Here's how the part is built. I have some questions about the finished solid (model axes, mm). A direction names the side the tool comes from. Coordinates: 2 decimals unless noted, no trailing zeros. Write each loop counter-clockwise with the first axis right and the second up, starting at its lowest first coordinate (ties: lowest second). Pieces come first, ordered by that corner, then holes.
```python
from build123d import *

# Parameters (mm, degrees)
BOSS_EXTRUDE1_DEPTH = 30
SKETCH2_R           = 11
CUT_EXTRUDE1_DEPTH  = 60
FILLET1_R           = 10
SKETCH3_R           = 2
CUT_EXTRUDE2_DEPTH  = 10
SKETCH13_R          = 13.5
CUT_EXTRUDE3_DEPTH  = 10


with BuildPart() as part:
    # Sketch1 → Boss-Extrude1 (new body, symmetric)
    with BuildSketch(Plane.XY):
        Polygon((-30, 30), (-30, -30), (30, -30), (30, 30), (24, 30), (24, -24.147945483), (-20, -24.147945483), (-20, 30), align=None)
    extrude(amount=BOSS_EXTRUDE1_DEPTH, both=True)

    # Sketch2 → Cut-Extrude1 (cut)
    with BuildSketch(Plane(origin=(0, 0, 0), x_dir=(0, 0, -1), z_dir=(1, 0, 0))):
        Circle(SKETCH2_R)
    extrude(amount=-CUT_EXTRUDE1_DEPTH, mode=Mode.SUBTRACT)

    # Fillet1
    fillet1_edges = [part.edges().sort_by_distance(p)[0] for p in [
        (-25, 30, -30),
        (27, 30, 30),
        (-25, 30, 30),
        (27, 30, -30),
    ]]
    fillet(fillet1_edges, radius=FILLET1_R)

    # Sketch3 → Cut-Extrude2 (cut, symmetric)
    with BuildSketch(Plane(origin=(0, -24.147945483, 0), x_dir=(1, 0, 0), z_dir=(0, 1, 0))):
        with Locations((-15, 22.5)):
            Circle(SKETCH3_R)
        with Locations((19, 22.5)):
            Circle(SKETCH3_R)
        with Locations((-15, -22.5)):
            Circle(SKETCH3_R)
        with Locations((19, -22.5)):
            Circle(SKETCH3_R)
    extrude(amount=CUT_EXTRUDE2_DEPTH, both=True, mode=Mode.SUBTRACT)

    # Sketch13 → Cut-Extrude3 (cut)
    with BuildSketch(Plane(origin=(30, 0, 0), x_dir=(0, 0, -1), z_dir=(1, 0, 0))):
        Circle(SKETCH13_R)
    extrude(amount=-CUT_EXTRUDE3_DEPTH, mode=Mode.SUBTRACT)


solid = part.part
```
1) Imagine slicing it at B-B on y = -19.5. Please give me the cut outline in (x, z).
Values follow:
outline: (-30, -30) - (-20, -30) - (-20, 30) - (-30, 30) - close; (24, -30) - (30, -30) - (30, 30) - (24, 30) - close
2) Imagine slicing it at C-C on z = 0. Please give me the cut outline in (x, y), then the cut area to 3 significant figures.
Values follow:
outline: (-30, -30) - (30, -30) - (30, -13.5) - (24, -13.5) - (24, -24.15) - (-20, -24.15) - (-20, -11) - (-30, -11) - close; (-30, 11) - (-20, 11) - (-20, 30) - (-30, 30) - close; (24, 13.5) - (30, 13.5) - (30, 30) - (24, 30) - close
area: 835 mm2
3) On a 3-axis mill with a long thin cutter (end or side, diameter ignored), from which of +Z, -Z, +X, -X, +Y, -Y can I reach the whole of each face in a straight line? I mean faces 4 (the face through (26.96, 26.99, 27.15)), 5 (the face through (2, -24.148, 0)), 6 (the face through (27.04, -13.18, 2.93)). Say none if no direction works.
Values follow:
face 4: +Z, +X, -X, +Y
face 5: +Z, -Z, +Y
face 6: +X
4) Will these pins go through, and if not, where does the flat tip stop? pin 1 (16 mm diameter, centred on y = 0, z = 0, fed in from -X); pin 2 (6.5 mm diameter, centred on x = -15, z = 22.5, fed in from +Y).
Values follow:
pin 1: passes through
pin 2: stops at y = -24.15
5) We'd pull the mould along Z, two halves only. Please class faces 1 (the face through (0, -30, 0)), 2 (the face through (26.96, 26.99, -27.15)), 3 (the face through (17.4, -27, -21.3)): pulls with the +Z half, pulls with the -Z half, needs draft (parallel to the pull), parting line crosses it, or undercut.
Values follow:
face 1: needs draft
face 2: pulls with the -Z half
face 3: undercut
6) Imagine slicing it at D-D on x = -25. Please give me the cut outline in (y, z).
Values follow:
outline: (-30, -30) - (20, -30) arc R10 ccw to (30, -20) - (30, 20) arc R10 ccw to (20, 30) - (-30, 30) - close; hole circle Ø22 at (0, 0)
7) Imagine slicing it at A-A on x = 19. Please give me the cut outline in (y, z).
Values follow:
outline: (-30, -30) - (-24.15, -30) - (-24.15, -24.5) - (-30, -24.5) - close; (-30, -20.5) - (-24.15, -20.5) - (-24.15, 20.5) - (-30, 20.5) - close; (-30, 24.5) - (-24.15, 24.5) - (-24.15, 30) - (-30, 30) - close
8) I need wall thicknesses on probe 1 along Z at (x, y) = (19, -27); probe 2 along X at (y, z) = (-25.6, 22.5); probe 3 along X at (y, z) = (-3.5, 21). Which ranges of each line are inside material? Lowest first, please.
Values follow:
probe 1: z = -30 to -24.5, -20.5 to 20.5, 24.5 to 30
probe 2: x = -30 to -17, -13 to 17, 21 to 30
probe 3: x = -30 to -20, 24 to 30
